Here's how the part is built. I have some questions about the finished solid (model axes, mm). A direction names the side the tool comes from. Give positions to 0.01 mm unless a question says otherwise; leave off trailing zeros. Order: outer loops, then holes, each group sorted by start corner. A loop starts at its lowest first (then second) coordinate and runs counter-clockwise, first axis right, second up. Notation, with made-up numbers: M 29,21.25 L 67,21.25 A15 ccw 67,45.25 Z; hole C -8,34 d2. An arc over 180 degrees is marked long. One line per item, written item: value. Start each with the question number.
from build123d import *

# Parameters (mm, degrees)
PAD_DEPTH    = 20
SKETCH001_W  = 21
SKETCH001_H  = 6.011268
PAD001_DEPTH = 16
POCKET_DEPTH = 13.006634
CHAMFER_SIZE = 10


with BuildPart() as part:
    # Sketch → Pad (new body)
    with BuildSketch(Plane.XY):
        Polygon((4.5, 6.5), (4.5, 10.5), (-4.5, 10.5), (-4.5, -10.5), (9.5, -10.5), (9.5, -6.5), (-0.5, -6.5), (-0.5, 6.5), align=None)
    extrude(amount=PAD_DEPTH)

    # Sketch001 (on Face3 of Pad) → Pad001 (join)
    with BuildSketch(Plane(origin=(-4.5, 0, 0), x_dir=(0, -1, 0), z_dir=(-1, 0, 0))):
        with Locations((0, 10)):
            Rectangle(SKETCH001_W, SKETCH001_H)
    extrude(amount=PAD001_DEPTH)

    # Sketch002 (on Face13 of Pad001) → Pocket (cut, through all)
    with BuildSketch(Plane(origin=(0, 0, 6.994366), x_dir=(1, 0, 0), z_dir=(0, 0, -1))):
        Polygon((-17.5, -10.5), (-12.5, -1.839746), (-7.5, -10.5), (-7.5, -16.27), (-17.5, -16.27), align=None)
    extrude(amount=-POCKET_DEPTH, mode=Mode.SUBTRACT)

    # Chamfer
    chamfer_edges = [part.edges().sort_by_distance(p)[0] for p in [
        (-20.5, -10.5, 10),
    ]]
    chamfer(chamfer_edges, length=CHAMFER_SIZE)


solid = part.part
Item 1: Will these pins go through, and if not, where does the flat tip stop? P1, Ø4.5, axis at y = 8, z = 10.5, coming from the +X side; P2, Ø8, axis at x = -11, y = 3, coming from the +Z side; P3, Ø4, axis at y = 0, z = 12.5, coming from the +X side.
Item 2: I want a section at B-B on y = -1.5. Write out the boundary of the cut face in (x, z), plus the area to 3 significant figures.
Item 3: Please list where these lines run through material, in increasing order: probe 1 along Y at (x, z) = (3.75, 7.5); probe 2 along X at (y, z) = (8, 14); probe 3 along X at (y, z) = (-4.5, 15). Write a range as [from, to].
Item 4: I want a section at A-A on z = 10.75. Write out the boundary of the cut face in (x, y), plus the area to 3 significant figures.
Item 5: For faces 1 (the face through (-11, 0, 6.994)), 2 (the face through (-0.5, 0, 10)), 3 (the face through (4.5, 8, 10)), 4 (the face through (-4.5, 0, 16)), 5 (the face through (-10.035, 6.109, 9.958)), which set-ups out of +Z, -Z, +X, -X, +Y, -Y let a thin tool reach every point of the face, with its end or its side?
Item 6: We'd pull the mould along Y, two halves only. Please class faces 6 (the face through (2, 6.5, 10)), 7 (the face through (-1, 0, 20)), 8 (the face through (0, 10.5, 10)): +Y half, -Y half, draft (parallel to the pull), parting line (faces both ways), or undercut.
Item 7: I want a section at C-C on y = 7.25. Write out the boundary of the cut face in (x, z).
Item 8: I want a section at D-D on z = 16. Write out the boundary of the cut face in (x, y).
Answer below:
1. P1: stops at x = 4.5
1. P2: stops at z = 13.01
1. P3: stops at x = -0.5
2. outline: M -19.5,6.99 L -4.5,6.99 L -4.5,0 L -0.5,0 L -0.5,20 L -4.5,20 L -4.5,13.01 L -19.5,13.01 Z
2. area: 170 mm²
3. probe 1: y = [-10.5, -6.5], [6.5, 10.5]
3. probe 2: x = [-4.5, 4.5]
3. probe 3: x = [-4.5, -0.5]
4. outline: M -20.5,-0.5 L -10.5,-10.5 L 9.5,-10.5 L 9.5,-6.5 L -0.5,-6.5 L -0.5,6.5 L 4.5,6.5 L 4.5,10.5 L -7.5,10.5 L -12.5,1.84 L -17.5,10.5 L -20.5,10.5 Z
4. area: 387 mm²
5. face 1: -Z, -X, +Y, -Y
5. face 2: +Z, -Z, +X
5. face 3: +Z, -Z, +X, +Y
5. face 4: +Z, -X, +Y, -Y
5. face 5: +Z, -Z, +Y
6. face 6: undercut
6. face 7: draft
6. face 8: +Y half
7. outline: M -20.5,6.99 L -15.62,6.99 L -15.62,13.01 L -20.5,13.01 Z; M -9.38,6.99 L -4.5,6.99 L -4.5,0 L 4.5,0 L 4.5,20 L -4.5,20 L -4.5,13.01 L -9.38,13.01 Z
8. outline: M -4.5,-10.5 L 9.5,-10.5 L 9.5,-6.5 L -0.5,-6.5 L -0.5,6.5 L 4.5,6.5 L 4.5,10.5 L -4.5,10.5 Z
